from build123d import *

# Parameters (mm, degrees)
SKETCH_1_R      = 1.5
SKETCH_1_R_2    = 3.5
EXTRUDE_1_DEPTH = 2
FILLET_1_R      = 0.5


with BuildPart() as part:
    # Эскиз1 → Бобышка-Вытянуть1 (new body)
    with BuildSketch(Plane(origin=(0, 0, 0), x_dir=(1, 0, 0), z_dir=(0, 1, 0))):
        with BuildLine():
            Line((-2.8125, 12.179484544), (-40.7875, 3.410255672))
            ThreePointArc((-40.7875, 3.410255672), (-43.5, 0), (-40.7875, -3.410255672))
            Line((-40.7875, -3.410255672), (-2.8125, -12.179484544))
            ThreePointArc((-2.8125, -12.179484544), (12.5, 0), (-2.8125, 12.179484544))
        make_face()
        with BuildLine():
            Line((-11.865804763, -3.930989356), (-28.888888889, 0))
            Line((-28.888888889, 0), (-11.865804763, 3.930989356))
            ThreePointArc((-11.865804763, 3.930989356), (-12.5, 0), (-11.865804763, -3.930989356))
        make_face(mode=Mode.SUBTRACT)
        with Locations((-40, 0)):
            Circle(SKETCH_1_R, mode=Mode.SUBTRACT)
        with Locations((5.833630945, 5.833630945)):
            Circle(SKETCH_1_R, mode=Mode.SUBTRACT)
        Circle(SKETCH_1_R_2, mode=Mode.SUBTRACT)
        with Locations((-5.833630945, -5.833630945)):
            Circle(SKETCH_1_R, mode=Mode.SUBTRACT)
        with Locations((5.833630945, -5.833630945)):
            Circle(SKETCH_1_R, mode=Mode.SUBTRACT)
        with Locations((-5.833630945, 5.833630945)):
            Circle(SKETCH_1_R, mode=Mode.SUBTRACT)
    extrude(amount=EXTRUDE_1_DEPTH)

    # Скругление1
    fillet_1_edges = [part.edges().sort_by_distance(p)[0] for p in [
        (-11.865804763, 1, -3.930989356),
        (-28.888888889, 1, 0),
        (-11.865804763, 1, 3.930989356),
    ]]
    fillet(fillet_1_edges, radius=FILLET_1_R)


solid = part.part
Part model, mm, in its own coordinate system. A direction names the side the tool comes from. Give positions to 0.01 mm unless a question says otherwise; leave off trailing zeros. Write each loop counter-clockwise with the first axis right and the second up, starting at its lowest first coordinate (ties: lowest second). Pieces come first, ordered by that corner, then holes.
1) Probe L1, parallel to X at y = 0.3, z = 0.25; L2, parallel to Z at x = 0, y = 1.6; L3, parallel to Z at x = -17, y = 0.6. List the from-to ranges inside material, lowest first.
Resolved:
L1: x = -43.49 to -41.48, -38.52 to -27.1, -12.5 to -3.49, 3.49 to 12.5
L2: z = -12.5 to -3.5, 3.5 to 12.5
L3: z = -8.9 to -2.75, 2.75 to 8.9
2) Cut at A-A on x = 0. Write the cut outline in (y, z).
Resolved:
outline: (0, -12.5) - (2, -12.5) - (2, -3.5) - (0, -3.5) - close; (0, 3.5) - (2, 3.5) - (2, 12.5) - (0, 12.5) - close
3) Cut at D-D on z = 5. Write the cut outline in (x, y).
Resolved:
outline: (-33.9, 0) - (-7.08, 0) - (-7.08, 2) - (-33.9, 2) - close; (-4.59, 0) - (4.59, 0) - (4.59, 2) - (-4.59, 2) - close; (7.08, 0) - (11.46, 0) - (11.46, 2) - (7.08, 2) - close
4) Cut at B-B on z = -2.5. Write the cut outline in (x, y).
Resolved:
outline: (-42.45, 0) - (-18.06, 0) - (-18.06, 2) - (-42.45, 2) - close; (-12.25, 0) - (-2.45, 0) - (-2.45, 2) - (-12.25, 2) - close; (2.45, 0) - (12.25, 0) - (12.25, 2) - (2.45, 2) - close
5) Two-plate mould, pull along X, no slides. Class faces 1 (the face through (12.496, 0.986, 0.315)), 2 (the face through (3.233, 0.986, 1.341)), 3 (the face through (-10, 2, 0)): released by +X, released by -X, zero draft, split by the parting line, or undercut.
Resolved:
face 1: split by the parting line
face 2: undercut
face 3: zero draft
6) Cut at C-C on y = 0.7. Write the cut outline in (x, z).
Resolved:
outline: (-40.79, -3.41) - (-2.81, -12.18) arc R12.5 ccw (long way) to (-2.81, 12.18) - (-40.79, 3.41) arc R3.5 ccw to start; hole circle Ø3 at (-40, 0); hole (-26.78, -0.49) - (-12.7, -3.74) arc R0.5 ccw to (-12.1, -3.13) arc R12.5 cw to (-12.1, 3.13) arc R0.5 ccw to (-12.7, 3.74) - (-26.78, 0.49) arc R0.5 ccw to start; hole circle Ø3 at (-5.83, -5.83); hole circle Ø3 at (-5.83, 5.83); hole circle Ø7 at (0, 0); hole circle Ø3 at (5.83, -5.83); hole circle Ø3 at (5.83, 5.83)
7) Pin check, flat tip, straight feed: pin 1 (2.5 mm diameter, centred on x = 5.83, z = -5.83, fed in from +Y). Stop position of the tip, or through.
Resolved:
pin 1: passes through
8) Which spindle directions (+Z, -Z, +X, -X, +Y, -Y) get a long thin tool onto all of the face, cutting with end or side? Do faces 4 (the face through (-10, 0, 0)), 5 (the face through (-19.8, 1, -2.1)). Say none if no direction does.
Resolved:
face 4: +Z, -Z, +X, -X, -Y
face 5: +Y, -Y
